```python
from build123d import *

# Parameters (mm, degrees)
SKETCH1_R           = 13.725
BOSS_EXTRUDE1_DEPTH = 32.6
SKETCH2_R           = 5
BOSS_EXTRUDE2_DEPTH = 3.62
SKETCH3_R           = 1.145
BOSS_EXTRUDE3_DEPTH = 11.43
BOSS_EXTRUDE4_START = 2.15
SKETCH4_R           = 5
BOSS_EXTRUDE4_DEPTH = 2.15
SKETCH5_R           = 1.15
BOSS_EXTRUDE5_DEPTH = 1
SKETCH6_W           = 3
SKETCH6_H           = 3.5
BOSS_EXTRUDE6_DEPTH = 5


with BuildPart() as part:
    # Sketch1 → Boss-Extrude1 (new body)
    with BuildSketch(Plane.XY):
        Circle(SKETCH1_R)
    extrude(amount=BOSS_EXTRUDE1_DEPTH)

    # Sketch2 → Boss-Extrude2 (add)
    with BuildSketch(Plane.XY.offset(32.6)):
        Circle(SKETCH2_R)
    extrude(amount=BOSS_EXTRUDE2_DEPTH)

    # Sketch3 → Boss-Extrude3 (add)
    with BuildSketch(Plane.XY.offset(36.22)):
        Circle(SKETCH3_R)
    extrude(amount=BOSS_EXTRUDE3_DEPTH)

    # Sketch4 → Boss-Extrude4 (add)
    with BuildSketch(Plane(origin=(0, 0, 0), x_dir=(-1, 0, 0), z_dir=(0, 0, -1)).offset(BOSS_EXTRUDE4_START)):
        with Locations(Location((0, 0, 0), (0, 0, 180))):
            Circle(SKETCH4_R)
    extrude(amount=-BOSS_EXTRUDE4_DEPTH)

    # Sketch5 → Boss-Extrude5 (add)
    with BuildSketch(Plane(origin=(0, 0, -2.15), x_dir=(-1, 0, 0), z_dir=(0, 0, -1))):
        Circle(SKETCH5_R)
    extrude(amount=BOSS_EXTRUDE5_DEPTH)

    # Sketch6 → Boss-Extrude6 (add)
    with BuildSketch(Plane(origin=(0, 0, 0), x_dir=(-1, 0, 0), z_dir=(0, 0, -1))):
        with Locations((-11.5, 0)):
            Rectangle(SKETCH6_W, SKETCH6_H)
        with Locations((11.5, 0)):
            Rectangle(SKETCH6_W, SKETCH6_H)
    extrude(amount=BOSS_EXTRUDE6_DEPTH)


solid = part.part
```
Part model, mm, in its own coordinate system. A direction names the side the tool comes from. Coordinates: 2 decimals unless noted, no trailing zeros. Order: outer loops, then holes, each group sorted by start corner. A loop starts at its lowest first (then second) coordinate and runs counter-clockwise, first axis right, second up. Notation, with made-up numbers: (37.5, -26.5) - (79.5, -26.5) arc R10 cw to (79.5, -19.5) - close; hole circle Ø8 at (23, 74.25). An arc over 180 degrees is marked (long way). Return JSON: item names as keys, results as strings. Group by question number.
Item 1: Which spindle directions (+Z, -Z, +X, -X, +Y, -Y) get a long thin tool onto all of the face, cutting with end or side? Do faces 5 (the face through (6, 0, 32.6)), 6 (the face through (-11, 1.75, -2)), 7 (the face through (-13, 0, -2)), 8 (the face through (12, -1.75, -2)), 9 (the face through (13, 0, -2)). Say none if no direction does.
Item 2: Cut at B-B (x = 0). List the corners of the cut face in (y, z) (3 decimals).
Item 3: Pin check, flat tips, straight feed: pin 1 (1.5 mm diameter, centred on x = -7, y = 5, fed in from -Z); pin 2 (1 mm diameter, centred on y = -0.5, z = -1.5, fed in from +X); pin 3 (2 mm diameter, centred on x = -7.5, z = 1, fed in from +Y). Stop position of each tip, or through.
Item 4: Cut at D-D (x = 3.5). List the corners of the cut face in (y, z), plus the area to 3 significant figures.
Item 5: Cut at C-C (z = 32). List the corners of the cut face in (x, y) (3 decimals).
Item 6: Drill centre lines: probe 1 along Z at (x, y) = (-7.25, 4.75); probe 2 along Y at (x, z) = (0.5, 0.5); probe 3 along Z at (x, y) = (12.5, -0.5). Where is each one in solid material? Low to high. Write a range as from..to.
Item 7: Pull direction X, two halves, no side cores. Call faces 1 (the face through (1, 1, -2.15)), 2 (the face through (1, -1, 36.22)), 3 (the face through (0, 0, -3.15)), 4 (the face through (1.092, 0.344, 41.855)): pulls with the +X half, pulls with the -X half, needs draft (parallel to the pull), parting line crosses it, or undercut.
Item 8: Cut at A-A (y = 0). List the corners of the cut face in (x, z) (3 decimals).
Check values:
{
 "1": {"face 5": "+Z", "face 6": "-Z, -X, +Y", "face 7": "-Z, -X, +Y, -Y", "face 8": "-Z, +X, -Y", "face 9": "-Z, +X, +Y, -Y"},
 "2": {"outline": "(-13.725, 0) - (-5, 0) - (-5, -2.15) - (-1.15, -2.15) - (-1.15, -3.15) - (1.15, -3.15) - (1.15, -2.15) - (5, -2.15) - (5, 0) - (13.725, 0) - (13.725, 32.6) - (5, 32.6) - (5, 36.22) - (1.145, 36.22) - (1.145, 47.65) - (-1.145, 47.65) - (-1.145, 36.22) - (-5, 36.22) - (-5, 32.6) - (-13.725, 32.6) - close"},
 "3": {"pin 1": "stops at z = 0", "pin 2": "stops at x = 13", "pin 3": "stops at y = 12.09"},
 "4": {"outline": "(-13.27, 0) - (-3.57, 0) - (-3.57, -2.15) - (3.57, -2.15) - (3.57, 0) - (13.27, 0) - (13.27, 32.6) - (3.57, 32.6) - (3.57, 36.22) - (-3.57, 36.22) - (-3.57, 32.6) - (-13.27, 32.6) - close", "area": "906 mm2"},
 "5": {"outline": "circle Ø27.45 at (0, 0)"},
 "6": {"probe 1": "z = 0..32.6", "probe 2": "y = -13.72..13.72", "probe 3": "z = -5..32.6"},
 "7": {"face 1": "undercut", "face 2": "needs draft", "face 3": "undercut", "face 4": "parting line crosses it"},
 "8": {"outline": "(-13.725, 0) - (-13, 0) - (-13, -5) - (-10, -5) - (-10, 0) - (-5, 0) - (-5, -2.15) - (-1.15, -2.15) - (-1.15, -3.15) - (1.15, -3.15) - (1.15, -2.15) - (5, -2.15) - (5, 0) - (10, 0) - (10, -5) - (13, -5) - (13, 0) - (13.725, 0) - (13.725, 32.6) - (5, 32.6) - (5, 36.22) - (1.145, 36.22) - (1.145, 47.65) - (-1.145, 47.65) - (-1.145, 36.22) - (-5, 36.22) - (-5, 32.6) - (-13.725, 32.6) - close"}
}
